Here's how the part is built. I have some questions about the finished solid (model axes, mm). A direction names the side the tool comes from. Give positions to 0.01 mm unless a question says otherwise; leave off trailing zeros. Write each loop counter-clockwise with the first axis right and the second up, starting at its lowest first coordinate (ties: lowest second). Pieces come first, ordered by that corner, then holes. Notation, with made-up numbers: M 32.5,-9.5 L 89.5,-9.5 A31 ccw 89.5,24.5 Z; hole C 26.5,77 d4. An arc over 180 degrees is marked long. Answer as CSV lines item,"result". Start each with the question number.
Q1. Suppose I cut it at C-C (z = 0.5). Write out the boundary of the cut face in (x, y), then the cut area to 3 significant figures.
Q2. On a 3-axis mill with a long thin cutter (end or side, diameter ignored), from which of +Z, -Z, +X, -X, +Y, -Y can I reach the whole of each face in a straight line? I mean faces 1 (the flat face through (-1, -21.2, 1)), 2 (the flat face through (-38.3, 0, 1)). Say none if no direction works.
Q3. Thinking about a two-plate mould opening in Y: for faces 3 (the cylindrical face through (-18.434, 18.985, 0.986)), 4 (the cylindrical face through (42.497, 20.059, 1.014)), 5 (the flat face through (-1, 14, 2)), which applies, +Y half, -Y half, draft (parallel to the pull), parting line (faces both ways), or undercut?
Q4. Suppose I cut it at B-B (x = -18.2). Write out the boundary of the cut face in (y, z).
Q5. Suppose I cut it at D-D (y = -1). Write out the boundary of the cut face in (x, z), then the cut area to 3 significant figures.
Q6. If I drill on line 1 along Y through (x, z) = (26.8, 1.55); line 2 along X through (y, z) = (1, 1.25); line 3 along X through (y, z) = (18, 0.7), over which ranges is the centre line in solid material (lowest first)?
Q7. Suppose I cut it at A-A (x = 15.5). Write out the boundary of the cut face in (y, z), then the cut area to 3 significant figures.
Q8. For pin 1 (6 mm diameter, centred on x = -5.5, y = -6, fed in from -Z), with a flat end and sliding along its axis, tell me the tip position at first contact or that it passes through.
```python
from build123d import *

# Parameters (mm, degrees)
SKETCH_W    = 87.4
SKETCH_H    = 42.4
SKETCH_R    = 1.8
SKETCH_W_2  = 76.6
SKETCH_H_2  = 21.8
PAD_DEPTH   = 2
FILLET_R    = 4
FILLET001_R = 1


with BuildPart() as part:
    # Sketch → Pad (new body)
    with BuildSketch(Plane.XY):
        Rectangle(SKETCH_W, SKETCH_H)
        with Locations((-18.2, 17.2)):
            Circle(SKETCH_R, mode=Mode.SUBTRACT)
        with Locations((-18.2, -17.2)):
            Circle(SKETCH_R, mode=Mode.SUBTRACT)
        with Locations((26.8, -17.2)):
            Circle(SKETCH_R, mode=Mode.SUBTRACT)
        with Locations((26.8, 17.2)):
            Circle(SKETCH_R, mode=Mode.SUBTRACT)
        Rectangle(SKETCH_W_2, SKETCH_H_2, mode=Mode.SUBTRACT)
    extrude(amount=PAD_DEPTH)

    # Fillet
    fillet_edges = [part.edges().sort_by_distance(p)[0] for p in [
        (43.7, -21.2, 1),
        (-43.7, -21.2, 1),
        (43.7, 21.2, 1),
        (-43.7, 21.2, 1),
    ]]
    fillet(fillet_edges, radius=FILLET_R)

    # Fillet001
    fillet001_edges = [part.edges().sort_by_distance(p)[0] for p in [
        (38.3, 10.9, 1),
        (38.3, -10.9, 1),
        (-38.3, -10.9, 1),
        (-38.3, 10.9, 1),
    ]]
    fillet(fillet001_edges, radius=FILLET001_R)


solid = part.part
```
Resolved:
1,outline,"M -43.7,-17.2 A4 ccw -39.7,-21.2 L 39.7,-21.2 A4 ccw 43.7,-17.2 L 43.7,17.2 A4 ccw 39.7,21.2 L -39.7,21.2 A4 ccw -43.7,17.2 Z; hole M -38.3,-9.9 A1 ccw -37.3,-10.9 L 37.3,-10.9 A1 ccw 38.3,-9.9 L 38.3,9.9 A1 ccw 37.3,10.9 L -37.3,10.9 A1 ccw -38.3,9.9 Z; hole C -18.2,-17.2 d3.6; hole C -18.2,17.2 d3.6; hole C 26.8,-17.2 d3.6; hole C 26.8,17.2 d3.6"
1,area,"1,980 mm^2"
2,face 1,"+Z, -Z, +X, -X, -Y"
2,face 2,"+Z, -Z"
3,face 3,"undercut"
3,face 4,"+Y half"
3,face 5,"draft"
4,outline,"M -21.2,0 L -19,0 L -19,2 L -21.2,2 Z; M -15.4,0 L -10.9,0 L -10.9,2 L -15.4,2 Z; M 10.9,0 L 15.4,0 L 15.4,2 L 10.9,2 Z; M 19,0 L 21.2,0 L 21.2,2 L 19,2 Z"
5,outline,"M -43.7,0 L -38.3,0 L -38.3,2 L -43.7,2 Z; M 38.3,0 L 43.7,0 L 43.7,2 L 38.3,2 Z"
5,area,"21.6 mm^2"
6,line 1,"-21.2 to -19, -15.4 to -10.9, 10.9 to 15.4, 19 to 21.2"
6,line 2,"-43.7 to -38.3, 38.3 to 43.7"
6,line 3,"-43.62 to -19.81, -16.59 to 25.19, 28.41 to 43.62"
7,outline,"M -21.2,0 L -10.9,0 L -10.9,2 L -21.2,2 Z; M 10.9,0 L 21.2,0 L 21.2,2 L 10.9,2 Z"
7,area,"41.2 mm^2"
8,pin 1,"through"
